from build123d import *

# Parameters (mm, degrees)
BOSS_EXTRUDE1_DEPTH = 7
SKETCH2_R           = 1.65
CUT_EXTRUDE1_DEPTH  = 8
CUT_EXTRUDE2_DEPTH  = 2
FILLET1_R           = 1


with BuildPart() as part:
    # Sketch1 → Boss-Extrude1 (new body)
    with BuildSketch(Plane.XY):
        Polygon((-2.750000021, 4.000000393), (5.249999979, 4.000000393), (10.750000021, 2), (12.750000021, 2), (12.750000021, -1.999999214), (10.750000021, -1.999999214), (5.249999979, -3.999999607), (-2.750000021, -3.999999607), (-12.750000021, -3.999999607), (-12.750000021, 4.000000393), align=None)
    extrude(amount=BOSS_EXTRUDE1_DEPTH)

    # Sketch2 → Cut-Extrude1 (cut)
    with BuildSketch(Plane(origin=(0, 4.000000393, 0), x_dir=(1, 0, 0), z_dir=(0, 1, 0))):
        with Locations((1.249999979, -3.5)):
            Circle(SKETCH2_R)
        with BuildLine():
            Line((-12.750000021, -2.5), (-2.051893418, -2.5))
            ThreePointArc((-2.051893418, -2.5), (1.249999979, -0.05), (4.551893375, -2.5))
            Line((4.551893375, -2.5), (12.750000021, -2.5))
            Line((12.750000021, -2.5), (12.750000021, 0))
            Line((12.750000021, 0), (-12.750000021, 0))
            Line((-12.750000021, 0), (-12.750000021, -2.5))
        make_face()
        with BuildLine():
            Line((-12.750000021, -5.5), (-1.561138581, -5.5))
            ThreePointArc((-1.561138581, -5.5), (1.249999979, -6.95), (4.061138538, -5.5))
            Line((4.061138538, -5.5), (12.750000021, -5.5))
            Line((12.750000021, -5.5), (12.750000021, -7))
            Line((12.750000021, -7), (-12.750000021, -7))
            Line((-12.750000021, -7), (-12.750000021, -5.5))
        make_face()
    extrude(amount=-CUT_EXTRUDE1_DEPTH, mode=Mode.SUBTRACT)

    # Sketch3 → Cut-Extrude2 (cut)
    with BuildSketch(Plane(origin=(12.750000021, 0, 0), x_dir=(0, 0, -1), z_dir=(1, 0, 0))):
        Polygon((-4, 2), (-2.6, 0), (-4, -2), (-2.5, -2), (-2.5, 0), (-2.5, 2), align=None)
    extrude(amount=-CUT_EXTRUDE2_DEPTH, mode=Mode.SUBTRACT)

    # Fillet1
    fillet1_edges = [part.edges().sort_by_distance(p)[0] for p in [
        (-7.40094672, 4.000000393, 2.5),
        (-7.40094672, -3.999999607, 2.5),
        (-12.750000021, 3.93e-07, 2.5),
        (-7.155569301, 4.000000393, 5.5),
        (-7.155569301, -3.999999607, 5.5),
        (-12.750000021, 3.93e-07, 5.5),
    ]]
    fillet(fillet1_edges, radius=FILLET1_R)


solid = part.part
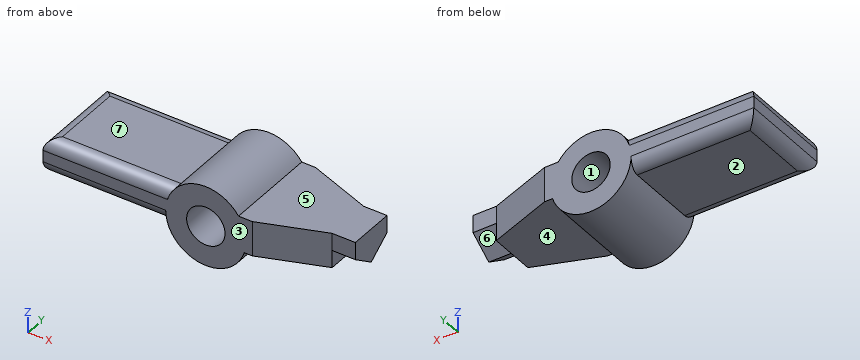
Can you work these out from the model? Positions are in its coordinate system, mm. Face numbers are marked on the shaded views. A direction names the side the tool comes from. Round coordinates to 2 decimals unless told otherwise and drop trailing zeros. Order: outer loops, then holes, each group sorted by start corner. A loop starts at its lowest first (then second) coordinate and runs counter-clockwise, first axis right, second up. Notation, with made-up numbers: (-3.75, 58) - (10.25, 58) arc R15 cw to (10.25, 74) - close; hole circle Ø7 at (58.25, 44.5). An arc over 180 degrees is marked (long way). Answer in a Markdown table with one row per item.
(1) Suppose I cut it at D-D, the plane z = 3. Please give me the cut outline in (x, y), plus the area to 3 significant figures.
From the geometry:
| item | result |
|---|---|
| outline | (-12.62, -3.87) - (-2.16, -3.87) - (-2.16, -4) - (-0.32, -4) - (-0.32, 4) - (-2.16, 4) - (-2.16, 3.87) - (-12.62, 3.87) - close; (2.82, -4) - (5.25, -4) - (10.75, -2) - (10.75, -0.57) - (12.75, -0.57) - (12.75, 0.57) - (10.75, 0.57) - (10.75, 2) - (5.25, 4) - (2.82, 4) - close |
| area | 150 mm2 |
(2) Suppose I cut it at A-A, the plane x = 1.25. Please give me the cut outline in (y, z), plus the area to 3 significant figures.
From the geometry:
| item | result |
|---|---|
| outline | (-4, 0.05) - (4, 0.05) - (4, 1.85) - (-4, 1.85) - close; (-4, 5.15) - (4, 5.15) - (4, 6.95) - (-4, 6.95) - close |
| area | 28.8 mm2 |
(3) Suppose I cut it at B-B, the plane x = -9.75. Please give me the cut outline in (y, z).
From the geometry:
| item | result |
|---|---|
| outline | (-4, 3.5) arc R1 ccw to (-3, 2.5) - (3, 2.5) arc R1 ccw to (4, 3.5) - (4, 4.5) arc R1 ccw to (3, 5.5) - (-3, 5.5) arc R1 ccw to (-4, 4.5) - close |
(4) Which directions (+Z, -Z, +X, -X, +Y, -Y) give clear straight access to the entire face, cutting with the end or side of a thin tool? Please do the marked faces 4, 5, 6 and 7.
From the geometry:
| item | result |
|---|---|
| face 4 | -Z, +X, +Y, -Y |
| face 5 | +Z, +X, +Y, -Y |
| face 6 | -Z, +X, +Y |
| face 7 | +Z, -X, +Y, -Y |
(5) For P1, Ø2, axis at x = 8, z = 2.5, coming from the -Y side; P2, Ø1.7, axis at x = 11.5, z = 5, coming from the -Y side; P3, Ø1.8, axis at x = -6.5, y = 1.5, coming from the -Z side, each with a flat end and sliding along its axis, tell me the tip position at first contact or that it passes through.
From the geometry:
| item | result |
|---|---|
| P1 | stops at y = -3.36 |
| P2 | stops at y = -2.04 |
| P3 | stops at z = 2.5 |
(6) Please list where these lines run through material, in increasing order: L1, parallel to X at y = 0.75, z = 3.5; L2, parallel to Z at x = 1.25, y = 0.5; L3, parallel to X at y = -1.75, z = 3.5. Write a range as from..to.
From the geometry:
| item | result |
|---|---|
| L1 | x = -12.75..-0.4, 2.9..12.75 |
| L2 | z = 0.05..1.85, 5.15..6.95 |
| L3 | x = -12.75..-0.4, 2.9..10.75 |
(7) Suppose I cut it at C-C, the plane y = -2.75. Please give me the cut outline in (x, z).
From the geometry:
| item | result |
|---|---|
| outline | (-12.75, 3.5) arc R1 ccw to (-11.75, 2.5) - (-2.05, 2.5) arc R3.45 ccw to (4.55, 2.5) - (8.69, 2.5) - (8.69, 5.5) - (4.06, 5.5) arc R3.45 ccw to (-1.56, 5.5) - (-11.75, 5.5) arc R1 ccw to (-12.75, 4.5) - close; hole circle Ø3.3 at (1.25, 3.5) |
(8) If we mould it in two halves opening along Z, with no side actions, what happens to the marked faces 1, 2 and 3? For each: released by +Z, released by -Z, zero draft, split by the parting line, or undercut.
From the geometry:
| item | result |
|---|---|
| face 1 | undercut |
| face 2 | released by -Z |
| face 3 | zero draft |
